from build123d import *

# Parameters (mm, degrees)
SKETCH1_W                        = 15.24
SKETCH1_H                        = 15.24
BOSS_EXTRUDE1_DEPTH              = 31.75
FILLET1_R                        = 0.79375
CUT_EXTRUDE1_DEPTH               = 16.24
SKETCH2_3_W                      = 15.24
SKETCH2_3_H                      = 7.9375
CUT_EXTRUDE2_DEPTH               = 6.35
F_4_0_209_DIAMETER_HOLE1_D       = 2.032
F_4_0_209_DIAMETER_HOLE1_DEPTH   = 6.35
F_4_0_209_DIAMETER_HOLE1_TIP     = 0.610474389
F_10_0_1935_DIAMETER_HOLE1_D     = 3.556
F_10_0_1935_DIAMETER_HOLE1_DEPTH = 6.35
F_10_0_1935_DIAMETER_HOLE1_TIP   = 1.068330181
FILLET2_R                        = 0.79375
FILLET3_R                        = 0.254


with BuildPart() as part:
    # Sketch1 → Boss-Extrude1 (new body)
    with BuildSketch(Plane(origin=(0, 0, 0), x_dir=(1, 0, 0), z_dir=(0, 1, 0))):
        Rectangle(SKETCH1_W, SKETCH1_H)
    extrude(amount=BOSS_EXTRUDE1_DEPTH)

    # Fillet1
    fillet1_edges = [part.edges().sort_by_distance(p)[0] for p in [
        (7.62, 15.875, 7.62),
        (-7.62, 15.875, 7.62),
        (-7.62, 15.875, -7.62),
        (7.62, 15.875, -7.62),
    ]]
    fillet(fillet1_edges, radius=FILLET1_R)

    # Sketch2 → Cut-Extrude1 (cut, through all)
    with BuildSketch(Plane.XY.offset(7.62)):
        with BuildLine():
            ThreePointArc((-7.62, 9.398), (-3.266426044, 12.7), (-7.62, 16.002))
            Line((-7.62, 16.002), (-7.62, 9.398))
        make_face()
    extrude(amount=-CUT_EXTRUDE1_DEPTH, mode=Mode.SUBTRACT)

    # Sketch2<3> → Cut-Extrude2 (cut)
    with BuildSketch(Plane.XY.offset(7.62)):
        with Locations((0, 27.78125)):
            Rectangle(SKETCH2_3_W, SKETCH2_3_H)
    extrude(amount=-CUT_EXTRUDE2_DEPTH, mode=Mode.SUBTRACT)

    # #4 (0.209) Diameter Hole1
    with Locations(Plane.XY.offset(1.27)):
        with Locations((0, 27.78125)):
            Hole(F_4_0_209_DIAMETER_HOLE1_D / 2, depth=F_4_0_209_DIAMETER_HOLE1_DEPTH)
            with Locations((0, 0, -(F_4_0_209_DIAMETER_HOLE1_DEPTH + F_4_0_209_DIAMETER_HOLE1_TIP / 2))):  # 118° drill point
                Cone(0, F_4_0_209_DIAMETER_HOLE1_D / 2, F_4_0_209_DIAMETER_HOLE1_TIP, mode=Mode.SUBTRACT)

    # #10 (0.1935) Diameter Hole1
    with Locations(Plane(origin=(0, 0, 0), x_dir=(-1, 0, 0), z_dir=(0, -1, 0))):
        with Locations((0, 0)):
            Hole(F_10_0_1935_DIAMETER_HOLE1_D / 2, depth=F_10_0_1935_DIAMETER_HOLE1_DEPTH)
            with Locations((0, 0, -(F_10_0_1935_DIAMETER_HOLE1_DEPTH + F_10_0_1935_DIAMETER_HOLE1_TIP / 2))):  # 118° drill point
                Cone(0, F_10_0_1935_DIAMETER_HOLE1_D / 2, F_10_0_1935_DIAMETER_HOLE1_TIP, mode=Mode.SUBTRACT)

    # Fillet2
    fillet2_edges = [part.edges().sort_by_distance(p)[0] for p in [
        (-7.387516008, 23.8125, 7.387516008),
        (7.387516008, 23.8125, 7.387516008),
        (-7.62, 23.8125, 4.048125),
        (-7.62, 27.78125, 1.27),
        (0, 23.8125, 7.62),
        (0, 23.8125, 1.27),
        (7.62, 23.8125, 4.048125),
        (7.62, 27.78125, 1.27),
    ]]
    fillet(fillet2_edges, radius=FILLET2_R)

    # Fillet3
    fillet3_edges = [part.edges().sort_by_distance(p)[0] for p in [
        (-7.387203478, 16.058494452, 7.387828364),
        (-7.387203478, 9.341505548, 7.387828364),
        (-7.62, 9.398, 0),
        (-7.387203472, 9.341505547, -7.387828369),
        (-7.387203472, 16.058494453, -7.387828369),
        (-3.266426044, 12.7, -7.62),
        (-7.62, 16.002, 0),
        (-3.266426044, 12.7, 7.62),
    ]]
    fillet(fillet3_edges, radius=FILLET3_R)


solid = part.part
Can you work these out from the model? Positions are in its coordinate system, mm. A direction names the side the tool comes from. Round coordinates to 2 decimals unless told otherwise and drop trailing zeros. Write each loop counter-clockwise with the first axis right and the second up, starting at its lowest first coordinate (ties: lowest second). Pieces come first, ordered by that corner, then holes. Notation, with made-up numbers: M 27,37.25 L 64,37.25 A18 ccw 64,48.25 Z; hole C 87.5,63 d5. An arc over 180 degrees is marked long. Use CSV: the item, a comma, the result in double quotes.
(1) I need wall thicknesses on line 1 along Z through (x, y) = (0, 2); line 2 along Y through (x, z) = (0, -2); line 3 along Z through (x, y) = (-6.5, 27). Which ranges of each line are inside material? Lowest first, please.
Check values:
line 1,"-7.62 to -1.78, 1.78 to 7.62"
line 2,"0 to 26.77, 28.8 to 31.75"
line 3,"-7.62 to 1.27"
(2) Imagine slicing it at C-C (z = -3.5). Write out the boundary of the cut face in (x, y), plus the area to 3 significant figures.
Check values:
outline,"M -7.62,0 L 7.62,0 L 7.62,31.75 L -7.62,31.75 L -7.62,16.32 A0.25 ccw -7.32,16.07 A3.43 cw long -7.32,9.33 A0.25 ccw -7.62,9.08 Z; hole C 0,27.78 d2.03"
area,"456 mm^2"
(3) Imagine slicing it at A-A (x = 5.75). Write out the boundary of the cut face in (y, z).
Check values:
outline,"M 0,-7.62 L 31.75,-7.62 L 31.75,1.27 L 24.61,1.27 A0.79 cw 23.81,2.06 L 23.81,6.83 A0.79 ccw 23.02,7.62 L 0,7.62 Z"
(4) Imagine slicing it at B-B (y = 12.7). Write out the boundary of the cut face in (x, z), plus the area to 3 significant figures.
Check values:
outline,"M -3.27,-7.37 A0.25 ccw -3.01,-7.62 L 6.83,-7.62 A0.79 ccw 7.62,-6.83 L 7.62,6.83 A0.79 ccw 6.83,7.62 L -3.01,7.62 A0.25 ccw -3.27,7.37 Z"
area,"166 mm^2"
(5) On a 3-axis mill with a long thin cutter (end or side, diameter ignored), from which of +Z, -Z, +X, -X, +Y, -Y can I reach the whole of each face in a straight line? I mean faces 5 (the cylindrical face through (-0.385, 3.219, 1.736)), 6 (the flat face through (0, 31.75, -3)), 7 (the flat face through (-7.62, 22, -1)), 8 (the cylindrical face through (0.13, 28.79, -1.95)), 9 (the flat face through (0, 29, 1.27)). Say none if no direction works.
Check values:
face 5,"-Y"
face 6,"+Z, -Z, +X, -X, +Y"
face 7,"+Z, -Z, -X, +Y, -Y"
face 8,"+Z"
face 9,"+Z, +X, -X, +Y"
(6) I'm going to push flat-ended pins straight in: pin 1 (2.5 mm diameter, centred on x = 2, z = 4, fed in from +Y); pin 2 (6 mm diameter, centred on x = -6.7, y = 12.7, fed in from +Z); pin 3 (2 mm diameter, centred on x = -3.5, y = 28, fed in from +Z). Where does each tip first touch, or does it pass through?
Check values:
pin 1,"y = 23.81"
pin 2,"through"
pin 3,"z = 1.27"
(7) We'd pull the mould along Z, two halves only. Please class faces 1 (the flat face through (-7.62, 4, 0)), 2 (the conical face through (-0.142, 7.233, 0.274)), 3 (the flat face through (0, 11, 7.62)), 4 (the flat face through (0, 16, -7.62)): +Z half, -Z half, draft (parallel to the pull), parting line (faces both ways), or undercut.
Check values:
face 1,"draft"
face 2,"undercut"
face 3,"+Z half"
face 4,"-Z half"
(8) Imagine slicing it at D-D (z = 6.5). Write out the boundary of the cut face in (x, y), plus the area to 3 significant figures.
Check values:
outline,"M -7.62,0 L 7.62,0 L 7.62,23.02 A0.79 ccw 6.83,23.81 L -6.83,23.81 A0.79 ccw -7.62,23.02 L -7.62,16.32 A0.25 ccw -7.32,16.07 A3.43 cw long -7.32,9.33 A0.25 ccw -7.62,9.08 Z"
area,"338 mm^2"
